Input: part model. Units: mm. Frame: model coordinates. A direction names the side the tool comes from. Coordinates: 2 decimals unless noted, no trailing zeros. Write each loop counter-clockwise with the first axis right and the second up, starting at its lowest first coordinate (ties: lowest second). Pieces come first, ordered by that corner, then holes. Notation, with made-up numbers: (26.5, 13) - (77.5, 13) arc R9 cw to (77.5, 21) - close; hole circle Ø2 at (76.25, 85.5). An arc over 180 degrees is marked (long way). One line per question, with ' | ' between items. Start each with the question number.
1) Section query B-B on x = 16.5. Give the number of separate pieces and of enclosed holes in the cut face, and give its area (3 significant figures).
2) Line query: line 1 (Z direction, x = 11, y = -10); line 2 (X direction, y = 1, z = -52); line 3 (X direction, y = -26, z = -75.5). Output: solid intervals per line, ascending.
3) First-contact query: P1, Ø4, axis at x = 3.5, y = -5.5, coming from the +Z side; P2, Ø1, axis at y = -23, z = 43, coming from the +X side; P3, Ø10, axis at y = -17.5, z = 1.5, coming from the +X side; P4, Ø1, axis at x = -8, y = -16, coming from the -Z side. Flat tips, straight axial feed; report the tip coordinate or a pass-through.
4) Draft query along Z for faces 1 (the cylindrical face through (30.996, 0.524, -1.68)), 2 (the flat face through (-1, 0, 80)), 3 (the flat face through (-1, 0, -75)). Return one class per face: released by +Z, released by -Z, zero draft, split by the parting line, or undercut.
5) Section query C-C on z = 47. Return loops of the section in (x, y), and give its area (3 significant figures).
6) Reachability of faces 4 (the flat face through (-30, 0, 78)), 5 (the flat face through (-2, 15, 78)), 6 (the flat face through (-1, 0, 75)), 7 (the flat face through (-1, 0, -80)) from +Z, -Z, +X, -X, +Y, -Y: full face, straight path, thin tool, end or side. Return the list, or none.
7) Section query A-A on x = -12.5. Return loops of the section in (y, z), and give its area (3 significant figures).
Autodesk Inventor part; units mm, degrees
ref_plane "XY Plane" through (0, 0, 0) normal (0, 0, 1) x (1, 0, 0)
sketch "Skizze1" plane through (0, 0, 0) normal (0, 0, 1) x (1, 0, 0)
  circle A0 centre (0, 0) radius 31
  circle A1 centre (0, 0) radius 29
  dimension "d0" = 62
  dimension "d1" = 58
extrude "Extrusion1" add sketch "Skizze1" along normal mid plane 300
sketch "Skizze2" plane through (0, 0, 0) normal (0, 1, 0) x (-1, 0, 0)
  line L0 (-11, 169.5773) -> (-11, -169.8146) construction
  line L1 (-74.8376, 0) -> (82.6362, 0) construction
  line L2 (-11, 75) -> (-11, -75)
  line L3 (-31, -150) -> (-31, 150)
  line L4 (31, 150) -> (-31, 150)
  line L5 (-31, -150) -> (31, -150)
  spline S0 degree 2 poles (-11, 75) (-17.8298, 136.4739) (-72.8449, 128.3193) knots 0 0 0 1 1 1
  spline S1 degree 2 poles (-11, -75) (-17.6171, -136.2673) (-74.8376, -130) knots 0 0 0 1 1 1
  line L6 (-72.8449, 128.3193) -> (-74.8376, -130)
  line L7 (-31, 120) -> (-31, 150)
  line L8 (-31, 150) -> (31, 150)
  line L9 (31, 150) -> (31, -150)
  line L10 (31, -150) -> (31, 150)
  line L11 (31, -150) -> (-31, -150)
  line L12 (-31, -150) -> (-31, -120)
  point P0 (0, 0)
  dimension "d4" = 11
  dimension "d5" = 150
  dimension "d6" = 30
  dimension "d7" = 30
extrude "Extrusion3" cut sketch "Skizze2" along normal mid plane 100 contours S0 L3 L4 L9 L5 S1 L2
ref_plane "Arbeitsebene3" through (0, 33.25, 0) normal (0, 1, 0) x (-1, 0, 0)
sketch "Skizze8" plane through (0, 33.25, 0) normal (0, 1, 0) x (-1, 0, 0)
  line L0 (-11, -75) -> (-11, 75)
  arc A0 (-11, 56.4646) -> (-14.2842, 92.4804) centre (-300.1138, 48.2584) ccw
  arc A1 (-11, 56.4646) -> (-14.2842, 92.4804) centre (-31.6354, 72.7405) ccw
  point P0 (0, 0)
extrude "Extrusion6" cut sketch "Skizze8" against normal blind 65
mirror "Spiegeln2" about plane through (0, 0, 0) normal (0, 0, 1) of "Extrusion6"
ref_plane "Arbeitsebene7" through (15, 0, 0) normal (1, 0, 0) x (0, 1, 0)
sketch "Skizze13" plane through (15, 0, 0) normal (1, 0, 0) x (0, 1, 0)
  line L0 (-18, 80) -> (-15, 80)
  line L1 (-15, 80) -> (-15, -80)
  line L2 (-15, -80) -> (-18, -80)
  line L3 (-18, -80) -> (-18, 80)
  line L4 (15, 80) -> (18, 80)
  line L5 (18, 80) -> (18, -80)
  line L6 (18, -80) -> (15, -80)
  line L7 (15, -80) -> (15, 80)
  line L8 (0, 161.0458) -> (0, -181.8657) construction
  line L9 (-78.3289, 0) -> (67.3027, 0) construction
  point P0 (0, 0)
  dimension "d66" = 30
  dimension "d67" = 3
  dimension "d68" = 3
  dimension "d69" = 160
extrude "Extrusion11" [suppressed]
sketch "Skizze14" plane through (15, 0, 0) normal (1, 0, 0) x (0, 1, 0)
  line L0 (-51.8177, 0) -> (40.0312, 0) construction
  line L1 (0, 87.1429) -> (0, -189.8015) construction
  line L2 (-15, 80) -> (15, 80)
  line L3 (15, 80) -> (15, 75)
  line L4 (15, 75) -> (-15, 75)
  line L5 (-15, 75) -> (-15, 80)
  line L6 (-15, -75) -> (15, -75)
  line L7 (15, -75) -> (15, -80)
  line L8 (15, -80) -> (-15, -80)
  line L9 (-15, -80) -> (-15, -75)
  point P0 (0, 0)
  dimension "d72" = 5
  dimension "d73" = 5
  dimension "d74" = 150
  dimension "d75" = 30
  dimension "d76" = 30
extrude "Extrusion12" add sketch "Skizze14" against normal blind 45
extrude "Extrusion13" add sketch "Skizze14" along normal blind 15
sketch "Skizze15" plane through (0, 0, 0) normal (0, 0, 1) x (1, 0, 0)
  circle A0 centre (0, 0) radius 31
  circle A1 centre (0, 0) radius 35.4738
extrude "Extrusion14" cut sketch "Skizze15" along normal mid plane 250
properties part number "_3D-Druck"
Answer key:
1) separate pieces: 4 | enclosed holes: 0 | area: 1,250 mm²
2) line 1: -80 to -75, 75 to 80 | line 2: 28.98 to 30.98 | line 3: 12.85 to 16.88
3) P1: z = 80 | P2: x = 21.32 | P3: x = 28.37 | P4: through
4) face 1: zero draft | face 2: released by +Z | face 3: undercut
5) outline: (11, -28.98) arc R31 ccw to (11, 28.98) - (11, 26.83) arc R29 cw to (11, -26.83) - close | area: 143 mm²
6) face 4: +Z, -Z, -X, +Y, -Y | face 5: +Z, -Z, -X | face 6: -X | face 7: -Z, -X
7) outline: (-15, -80) - (15, -80) - (15, -75) - (-15, -75) - close; (-15, 75) - (15, 75) - (15, 80) - (-15, 80) - close | area: 300 mm²
